The listing builds one solid part. Answer for the finished solid, in the listing's coordinates (mm). Face numbers are marked on the shaded views. Coordinates: 2 decimals unless noted, no trailing zeros. Answer as CSV lines item,"result".
```python
from build123d import *

# Parameters (mm, degrees)
F0_R     = 2.1
F0_W     = 2.462149
F0_H     = 1.64
F0_W_2   = 2.954578
F0_W_3   = 2.554638
F0_W_4   = 2.751813
F0_W_5   = 2.700622
F0_W_6   = 3.026464
F0_W_7   = 2.722847
F0_W_8   = 2.821042
F1_DEPTH = 200


with BuildPart() as f1:
    # F0 (on Front) → F1 (new body)
    with BuildSketch(Plane.XZ):
        Polygon((30, 4.555675), (30, 10), (24.22707, 10), (22.920883, 8.2), (24.930604, 8.2), (28.2, 8.2), (28.2, 4.884325), (28.2, 2.928185), align=None)
        Polygon((28.2, 8.2), (24.930604, 8.2), (24.930604, 6.56), (26.56, 6.56), (26.56, 4.884325), (28.2, 4.884325), align=None)
        Polygon((26.56, 6.56), (24.930604, 6.56), (21.376314, 2.85), (22.85, 2.85), (22.85, 1.029287), (26.56, 4.884325), align=None)
        Polygon((28.2, -4.97699), (26.56, -4.97699), (26.56, -6.56), (24.907887, -6.56), (24.907887, -8.2), (28.2, -8.2), align=None)
        Polygon((28.2, -2.827582), (28.2, -4.97699), (28.2, -8.2), (24.907887, -8.2), (22.780269, -8.2), (24.227049, -10), (30, -10), (30, -3.998783), align=None)
        Polygon((26.56, -4.97699), (22.85, -1.368018), (22.85, -2.85), (21.271573, -2.85), (24.907887, -6.56), (26.56, -6.56), align=None)
        Polygon((22.85, 2.85), (21.376314, 2.85), (18.752582, 2.85), (17.15, 2.85), (17.15, 1.181537), (17.15, -1.454411), (17.15, -2.85), (18.781548, -2.85), (21.271573, -2.85), (22.85, -2.85), (22.85, -1.368018), (22.85, 1.029287), align=None)
        with Locations((20, 0)):
            Circle(F0_R, mode=Mode.SUBTRACT)
        Polygon((17.15, 2.85), (18.752582, 2.85), (14.610378, 6.56), (12.148229, 6.56), (17.15, 1.181537), align=None)
        with Locations((13.379303, 7.38)):
            Rectangle(F0_W, F0_H)
        Polygon((12.148229, 8.2), (14.610378, 8.2), (17.26873, 8.2), (15.720541, 10), (4.219369, 10), (2.896034, 8.2), (5.051448, 8.2), (8.006026, 8.2), align=None)
        with Locations((6.528737, 7.38)):
            Rectangle(F0_W_2, F0_H)
        Polygon((2.85, 1.123604), (8.006026, 6.56), (5.051448, 6.56), (1.343741, 2.85), (2.85, 2.85), align=None)
        Polygon((17.15, -2.85), (17.15, -1.454411), (12.577136, -6.56), (15.131774, -6.56), (18.781548, -2.85), align=None)
        with Locations((13.854455, -7.38)):
            Rectangle(F0_W_3, F0_H)
        Polygon((15.131774, -8.2), (12.577136, -8.2), (8.006026, -8.2), (5.254213, -8.2), (2.818424, -8.2), (4.436373, -10), (15.602568, -10), (17.118241, -8.2), align=None)
        with Locations((6.63012, -7.38)):
            Rectangle(F0_W_4, F0_H)
        Polygon((5.254213, -6.56), (8.006026, -6.56), (2.85, -1.106813), (2.85, -2.85), (1.51754, -2.85), align=None)
        Polygon((2.85, -1.106813), (2.85, 1.123604), (2.85, 2.85), (1.343741, 2.85), (-1.308073, 2.85), (-2.85, 2.85), (-2.85, 1.129449), (-2.85, -1.540485), (-2.85, -2.85), (-1.461518, -2.85), (1.51754, -2.85), (2.85, -2.85), align=None)
        Circle(F0_R, mode=Mode.SUBTRACT)
        Polygon((-2.85, 2.85), (-1.308073, 2.85), (-4.837296, 6.56), (-7.537918, 6.56), (-2.85, 1.129449), align=None)
        with Locations((-6.187607, 7.38)):
            Rectangle(F0_W_5, F0_H)
        Polygon((-7.537918, 8.2), (-4.837296, 8.2), (-2.768134, 8.2), (-4.417359, 10), (-15.527925, 10), (-17.283811, 8.2), (-14.860827, 8.2), (-11.834363, 8.2), align=None)
        with Locations((-13.347595, 7.38)):
            Rectangle(F0_W_6, F0_H)
        Polygon((-17.15, 1.267669), (-11.834363, 6.56), (-14.860827, 6.56), (-18.599909, 2.85), (-17.15, 2.85), align=None)
        Polygon((-5.086812, -6.56), (-1.461518, -2.85), (-2.85, -2.85), (-2.85, -1.540485), (-7.809659, -6.56), align=None)
        with Locations((-6.448236, -7.38)):
            Rectangle(F0_W_7, F0_H)
        Polygon((-2.881428, -8.2), (-5.086812, -8.2), (-7.809659, -8.2), (-12.576681, -8.2), (-15.397723, -8.2), (-17.08678, -8.2), (-15.658125, -10), (-4.417359, -10), align=None)
        with Locations((-13.987202, -7.38)):
            Rectangle(F0_W_8, F0_H)
        Polygon((-15.397723, -6.56), (-12.576681, -6.56), (-17.15, -1.227868), (-17.15, -2.85), (-18.736489, -2.85), align=None)
        Polygon((-17.15, -1.227868), (-17.15, 1.267669), (-17.15, 2.85), (-18.599909, 2.85), (-21.29855, 2.85), (-22.85, 2.85), (-22.85, 1.455018), (-22.85, -1.113568), (-22.85, -2.85), (-21.168495, -2.85), (-18.736489, -2.85), (-17.15, -2.85), align=None)
        with Locations((-20, 0)):
            Circle(F0_R, mode=Mode.SUBTRACT)
        Polygon((-22.85, 2.85), (-21.29855, 2.85), (-25.195252, 6.56), (-26.56, 6.56), (-26.56, 5.266924), (-22.85, 1.455018), align=None)
        Polygon((-24.907576, -6.56), (-21.168495, -2.85), (-22.85, -2.85), (-22.85, -1.113568), (-26.56, -5.145273), (-26.56, -6.56), align=None)
        Polygon((-26.56, 6.56), (-25.195252, 6.56), (-25.195252, 8.2), (-28.2, 8.2), (-28.2, 5.266924), (-26.56, 5.266924), align=None)
        Polygon((-28.2, 8.2), (-25.195252, 8.2), (-22.697506, 8.2), (-24.213179, 10), (-30, 10), (-30, 4.390912), (-28.2, 2.696034), (-28.2, 5.266924), align=None)
        Polygon((-24.907576, -8.2), (-24.907576, -6.56), (-26.56, -6.56), (-26.56, -5.145273), (-28.2, -5.145273), (-28.2, -8.2), align=None)
        Polygon((-23.055149, -8.2), (-24.907576, -8.2), (-28.2, -8.2), (-28.2, -5.145273), (-28.2, -2.76243), (-30, -4.472366), (-30, -10), (-24.772262, -10), align=None)
    extrude(amount=F1_DEPTH)


solid = f1.part
```
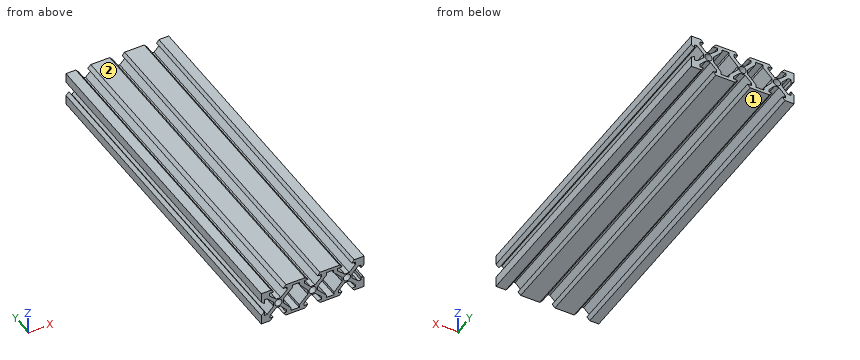
Q1. Find section A-A (y = -29). Count the separate pieces of the cut face and the enclosed holes in it, and give its area (3 significant figures).
Output:
separate pieces,"1"
enclosed holes,"5"
area,"435 mm2"
Q2. Flat-ended cylindrical pins translate along their axes: pin 1 Ø0.7 at (x, y) = (-3.5, -65) entering from +Z; pin 2 Ø1.3 at (y, z) = (-99.5, -0.5) entering from -X; pin 3 Ø1.5 at (x, y) = (-23.5, -51) entering from -Z. Find the tip coordinate at first contact, or state that the pin passes through.
Output:
pin 1,"z = 9.38"
pin 2,"x = -22.88"
pin 3,"z = -9.45"
Q3. Straight lines are drawn through the part: line 1 (Z direction, x = 20, y = -58); line 2 (Z direction, x = 11.5, y = -109); line 3 (Z direction, x = -24.5, y = -170). For each, find the intervals that lie inside material, in ascending order.
Output:
line 1,"-2.85 to -2.1, 2.1 to 2.85"
line 2,"-10 to -8.2, 8.2 to 10"
line 3,"-9.71 to -8.2, -6.16 to -2.91, 3.15 to 5.9, 8.2 to 10"
Q4. The mould has two halves that part along Z. Classify the marked faces 1 and 2: pulls with the +Z half, pulls with the -Z half, needs draft (parallel to the pull), parting line crosses it, or undercut.
Output:
face 1,"pulls with the -Z half"
face 2,"pulls with the +Z half"
